Print and shaded views of the part. All mm, measured from the part's lowest x, y and z. Coordinates: 2 decimals unless noted, no trailing zeros. Order: outer loops, then holes, each group sorted by start corner. A loop starts at its lowest first (then second) coordinate and runs counter-clockwise, first axis right, second up. Notation, with made-up numbers: M 15,-9.5 L 55,-9.5 A24 cw 55,15.5 Z; hole C 28,-40 d2. An arc over 180 degrees is marked long. Return JSON: item names as keys, results as strings.
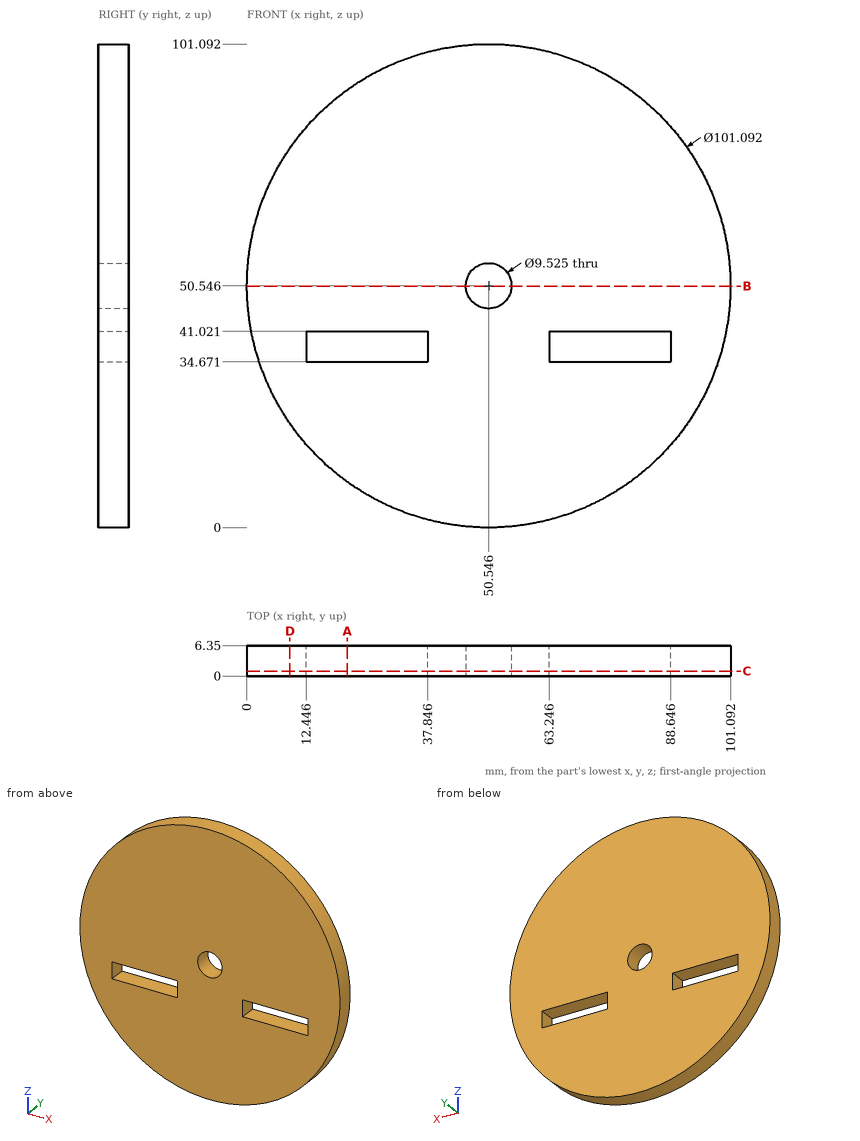
Item 1: Wall check: line 1 (X direction, y = 5.75, z = 48); line 2 (Z direction, x = 48.5, y = 4.75); line 3 (X direction, y = 1.25, z = 39). Give the ranges that are in metal, low to high.
Check result:
{"line 1": "x = 0.06 to 46.52, 54.57 to 101.03", "line 2": "z = 0.04 to 46.25, 54.85 to 101.05", "line 3": "x = 1.34 to 12.45, 37.85 to 63.25, 88.65 to 99.76"}
Item 2: Drop flat-ended pins along their axis: pin 1 Ø3 at (x, y) = (31.5, 4) entering from +Z; pin 2 Ø1 at (x, y) = (52.5, 2) entering from -Z; pin 3 Ø1.9 at (x, y) = (78.5, 3.5) entering from -Z; pin 4 Ø2 at (x, z) = (16, 62) entering from -Y. Give the stop position or say it passes through.
Check result:
{"pin 1": "stops at z = 97.95", "pin 2": "stops at z = 0.02", "pin 3": "stops at z = 7.82", "pin 4": "stops at y = 0"}
Item 3: Saw through at A-A (x = 21). Write the cut outline in (y, z).
Check result:
{"outline": "M 0,9.53 L 6.35,9.53 L 6.35,34.67 L 0,34.67 Z; M 0,41.02 L 6.35,41.02 L 6.35,91.56 L 0,91.56 Z"}
Item 4: Saw through at C-C (y = 1). Write the cut outline in (x, z) (1 decimal).
Check result:
{"outline": "C 50.5,50.5 d101.1; hole M 12.4,34.7 L 37.8,34.7 L 37.8,41 L 12.4,41 Z; hole C 50.5,50.5 d9.5; hole M 63.2,34.7 L 88.6,34.7 L 88.6,41 L 63.2,41 Z"}
Item 5: Saw through at D-D (x = 9). Write the cut outline in (y, z), and give its area (3 significant figures).
Check result:
{"outline": "M 0,21.76 L 6.35,21.76 L 6.35,79.34 L 0,79.34 Z", "area": "366 mm2"}
Item 6: Saw through at B-B (z = 50.5). Write the cut outline in (x, y).
Check result:
{"outline": "M 0,0 L 45.78,0 L 45.78,6.35 L 0,6.35 Z; M 55.31,0 L 101.09,0 L 101.09,6.35 L 55.31,6.35 Z"}
